from build123d import *

# Parameters (mm, degrees)
BOSS_EXTRUDE1_DEPTH            = 12.7
SKETCH2_R                      = 3.175
CUT_EXTRUDE1_DEPTH             = 62.233889922
SKETCH3_W                      = 6.35
SKETCH3_H                      = 11.43
CUT_EXTRUDE2_DEPTH             = 97.151665612
SKETCH4_R                      = 4
CUT_EXTRUDE3_DEPTH             = 62.233889922
SKETCH5_R                      = 1
CUT_EXTRUDE4_DEPTH             = 62.233889922
SKETCH6_W                      = 6.35
SKETCH6_H                      = 11.43
CUT_EXTRUDE5_DEPTH             = 61.238042589
M2X0_4_TAPPED_HOLE1_AT_2_COUNT = 2
M2X0_4_TAPPED_HOLE1_AT_2_PITCH = 5.334


with BuildPart() as part:
    # Sketch1 → Boss-Extrude1 (new body)
    with BuildSketch(Plane.XY):
        Polygon((-42.800130549, -5.715), (-10.39539802, -41.91), (10.39539802, -41.91), (42.800130549, -5.715), (42.800130549, 5.715), (-42.800130549, 5.715), align=None)
    extrude(amount=-BOSS_EXTRUDE1_DEPTH)

    # Sketch2 → Cut-Extrude1 (cut, through all)
    with BuildSketch(Plane.XY):
        Circle(SKETCH2_R)
    extrude(amount=-CUT_EXTRUDE1_DEPTH, mode=Mode.SUBTRACT)

    # Sketch3 → Cut-Extrude2 (cut, through all)
    with BuildSketch(Plane(origin=(42.800130549, 0, 0), x_dir=(0, 0, -1), z_dir=(1, 0, 0))):
        with Locations((9.525, 0)):
            Rectangle(SKETCH3_W, SKETCH3_H)
    extrude(amount=-CUT_EXTRUDE2_DEPTH, mode=Mode.SUBTRACT)

    # Sketch4 → Cut-Extrude3 (cut, through all)
    with BuildSketch(Plane.XY):
        with Locations((0, -15.24)):
            Circle(SKETCH4_R)
    extrude(amount=-CUT_EXTRUDE3_DEPTH, mode=Mode.SUBTRACT)

    # Sketch5 → Cut-Extrude4 (cut, through all)
    with BuildSketch(Plane.XY):
        with Locations((39.625130549, 3.175)):
            Circle(SKETCH5_R)
        with Locations((39.625130549, -3.175)):
            Circle(SKETCH5_R)
    cut_extrude4 = extrude(amount=-CUT_EXTRUDE4_DEPTH, mode=Mode.SUBTRACT)

    # Mirror1: Cut-Extrude4 across plane
    add(cut_extrude4.mirror(Plane(origin=(0, 0, 0), x_dir=(0, 0, 1), z_dir=(1, 0, 0))), mode=Mode.SUBTRACT)

    # Sketch6 → Cut-Extrude5 (cut, through all)
    with BuildSketch(Plane(origin=(0, 0, -6.35), x_dir=(-1, 0, 0), z_dir=(0, 0, -1))):
        with Locations((-39.625130549, 0)):
            Rectangle(SKETCH6_W, SKETCH6_H)
        with Locations((39.625130549, 0)):
            Rectangle(SKETCH6_W, SKETCH6_H)
    extrude(amount=-CUT_EXTRUDE5_DEPTH, mode=Mode.SUBTRACT)

    # Sketch8 → M2x0.4 Tapped Hole1 (revolve, cut)
    with BuildSketch(Plane(origin=(-36.450130549, 2.667, -3.175), x_dir=(0, 0, 1), z_dir=(0, 1, 0))):
        Polygon((0, 0), (0, 5.814688495), (0.8, 5.334), (0.8, 0), align=None)
    m2x0_4_tapped_hole1 = revolve(axis=Axis((-42.800130549, 2.667, -3.175), (1, 0, 0)), mode=Mode.SUBTRACT)

    # M2x0.4 Tapped Hole1 at 2: M2x0.4 Tapped Hole1 ×2
    with Locations(*[(0, -i * M2X0_4_TAPPED_HOLE1_AT_2_PITCH, 0) for i in range(1, M2X0_4_TAPPED_HOLE1_AT_2_COUNT)]):
        add(m2x0_4_tapped_hole1, mode=Mode.SUBTRACT)

    # Mirror2: M2x0.4 Tapped Hole1 across plane
    add(m2x0_4_tapped_hole1.mirror(Plane(origin=(0, 0, 0), x_dir=(0, 0, 1), z_dir=(1, 0, 0))), mode=Mode.SUBTRACT)

    # Mirror2 copy 1 sketch → Mirror2 copy 1 (revolve, cut)
    with BuildSketch(Plane(origin=(36.450130549, -2.667, -3.175), x_dir=(0, 0, 1), z_dir=(0, 1, 0))):
        Polygon((0, 0), (0, -5.814688495), (0.8, -5.334), (0.8, 0), align=None)
    revolve(axis=Axis((42.800130549, -2.667, -3.175), (1, 0, 0)), mode=Mode.SUBTRACT)


solid = part.part
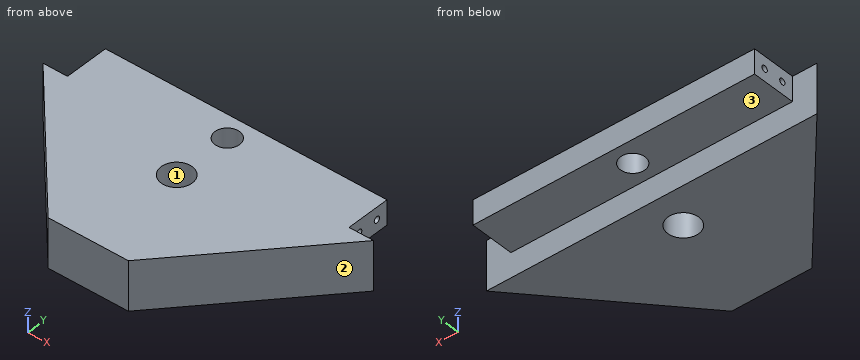
Work out the finished part from the listing and answer in its coordinate system (mm). Face numbers are marked on the shaded views. Give positions to 0.01 mm unless a question says otherwise; leave off trailing zeros. Order: outer loops, then holes, each group sorted by start corner. A loop starts at its lowest first (then second) coordinate and runs counter-clockwise, first axis right, second up. Notation, with made-up numbers: (87.25, 7) - (129.25, 7) arc R13 cw to (129.25, 11) - close; hole circle Ø1 at (35.25, 23). An arc over 180 degrees is marked (long way). Answer as CSV lines item,"result". Start each with the question number.
Q1. The part is cut by section D-D (z = -5). Write down the section's boundary in (x, y) (3 decimals).
Q2. Find the intervals of material crossed by L1, parallel to Y at x = -6.5, z = -7 (3 decimals); L2, parallel to X at y = 3.5, z = -3.25; L3, parallel to Z at x = 13, y = -3, in increasing order. Write a range as [from, to].
Q3. The part is cut by section C-C (z = -8.5). Write down the section's boundary in (x, y) (3 decimals), then the cut area to 3 significant figures.
Q4. The part is cut by section A-A (x = 0). Write down the section's boundary in (y, z) (3 decimals), then the cut area to 3 significant figures.
Q5. The mould has two halves that part along Y. Classify the marked faces 1, 2 and 3: +Y half, -Y half, draft (parallel to the pull), parting line (faces both ways), or undercut.
Q6. The part is cut by section B-B (y = 0). Write down the section's boundary in (x, z) (3 decimals), then the cut area to 3 significant figures.
Q7. Given pin 1 Ø1 at (y, z) = (-2.667, -3.175) entering from -X; pin 2 Ø3 at (y, z) = (-20.5, -6) entering from +X; pin 3 Ø2.5 at (y, z) = (2.667, -3.175) entering from -X, each flat-ended and moving along its own axis, determine where each tip first touches the part or whether it passes through.
Check result:
1,outline,"(-42.8, -5.715) - (-10.395, -41.91) - (10.395, -41.91) - (42.8, -5.715) - (36.45, -5.715) - (36.45, 5.715) - (-36.45, 5.715) - (-36.45, -5.715) - close; hole circle Ø8 at (0, -15.24); hole circle Ø6.35 at (0, 0)"
2,L1,"y = [-41.91, -5.715]"
2,L2,"x = [-36.45, 36.45]"
2,L3,"z = [-6.35, 0]"
3,outline,"(-42.8, -5.715) - (-10.395, -41.91) - (10.395, -41.91) - (42.8, -5.715) - close; hole circle Ø8 at (0, -15.24)"
3,area,"1,880 mm²"
4,outline,"(-41.91, -12.7) - (-19.24, -12.7) - (-19.24, 0) - (-41.91, 0) - close; (-11.24, -12.7) - (-5.715, -12.7) - (-5.715, -6.35) - (-3.175, -6.35) - (-3.175, 0) - (-11.24, 0) - close; (3.175, -6.35) - (5.715, -6.35) - (5.715, 0) - (3.175, 0) - close"
4,area,"390 mm²"
5,face 1,"undercut"
5,face 2,"-Y half"
5,face 3,"draft"
6,outline,"(-36.45, -6.35) - (-3.175, -6.35) - (-3.175, 0) - (-36.45, 0) - close; (3.175, -6.35) - (36.45, -6.35) - (36.45, 0) - (3.175, 0) - close"
6,area,"423 mm²"
7,pin 1,"stops at x = -30.94"
7,pin 2,"stops at x = 30.91"
7,pin 3,"stops at x = -36.45"
